Read the model definition and answer for the solid it produces. Units are mm, in the model's axes. Round coordinates to 2 decimals unless told otherwise and drop trailing zeros. Write each loop counter-clockwise with the first axis right and the second up, starting at its lowest first coordinate (ties: lowest second). Pieces come first, ordered by that corner, then holes.
from build123d import *

# Parameters (mm, degrees)
F0_W            = 139.7
F0_H            = 3.175
F1_DEPTH        = 50.8
F3_D            = 3.3
F4_W            = 38.1
F4_H            = 38.1
F5_DEPTH        = 3.176
F7_D            = 2.2606
F9_D            = 2.7051
F11_D           = 2.2606
F13_D           = 4.9784
F13_CSINK_D     = 9.1186
F13_CSINK_ANGLE = 82


with BuildPart() as f1:
    # F0 (on Front) → F1 (new body, symmetric)
    with BuildSketch(Plane.XZ):
        with Locations((-69.85, 1.5875)):
            Rectangle(F0_W, F0_H)
    extrude(amount=F1_DEPTH, both=True)

    # F3 (through all)
    with Locations(Plane.XY.offset(3.175)):
        with Locations((-78.994, 4.572), (-78.994, -4.572), (-89.154, 0), (-109.22, 0), (-119.38, 4.572), (-119.38, -4.572)):
            Hole(F3_D / 2)

    # F4 (on face) → F5 (cut, through all)
    with BuildSketch(Plane.XY.offset(3.175)):
        with Locations((-19.05, 31.75)):
            Rectangle(F4_W, F4_H)
    extrude(amount=-F5_DEPTH, mode=Mode.SUBTRACT)

    # F7 (through all)
    with Locations(Plane.XY.offset(3.175)):
        with Locations((-26.9875, -44.45), (-26.9875, -19.05), (-4.7625, -19.05), (-4.7625, -44.45)):
            Hole(F7_D / 2)

    # F9 (through all)
    with Locations(Plane.XY.offset(3.175)):
        with Locations((-86.36, 11.43), (-66.36, 11.43)):
            Hole(F9_D / 2)

    # F11 (through all)
    with Locations(Plane.XY.offset(3.175)):
        with Locations((-135.382, -2.54), (-98.298, -2.54), (-98.298, 22.225), (-135.382, 22.225)):
            Hole(F11_D / 2)

    # F13 (through all)
    with Locations(Plane(origin=(0, 0, 0), x_dir=(1, 0, 0), z_dir=(0, 0, -1))):
        with Locations((-30.1625, 31.75)):
            CounterSinkHole(F13_D / 2, F13_CSINK_D / 2, counter_sink_angle=F13_CSINK_ANGLE)


solid = f1.part
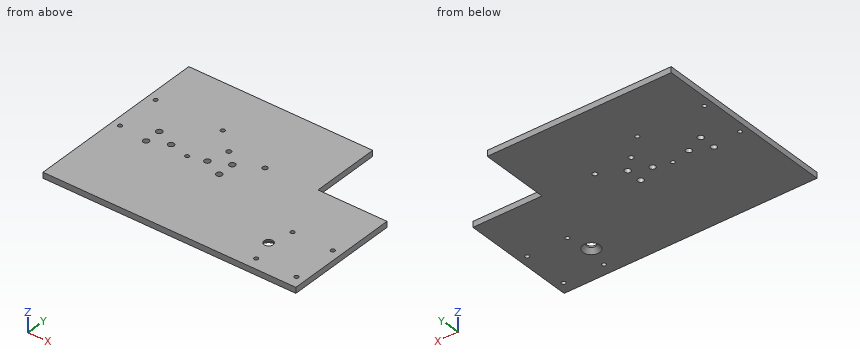
Q1. Section D-D (z = 0.7) is taken. State how many separate pieces and enclosed holes the cut face has, then the cut area to 3 significant figures.
Verdict:
separate pieces: 1
enclosed holes: 17
area: 12,600 mm2
Q2. Straight lines are drawn through the part: probe 1 along X at (y, z) = (22.5, 1.45); probe 2 along X at (y, z) = (-1, 2.1); probe 3 along Y at (x, z) = (-24.5, 1.85). For each, find the intervals that lie inside material, in ascending order.
Verdict:
probe 1: x = -139.7 to -136.48, -134.29 to -99.39, -97.2 to -38.1
probe 2: x = -139.7 to -110.53, -107.91 to -90.47, -87.84 to 0
probe 3: y = -50.8 to 12.7
Q3. Flat-ended cylindrical pins translate along their axes: pin 1 Ø2 at (x, y) = (-119.38, 4.572) entering from +Z; pin 2 Ø5.5 at (x, y) = (-89.154, 0) entering from -Z. Find the tip coordinate at first contact, or state that the pin passes through.
Verdict:
pin 1: passes through
pin 2: stops at z = 0
Q4. Section B-B (x = -109.22) is taken. Determine the outline of the cut face in (y, z) (3 decimals), then the cut area to 3 significant figures.
Verdict:
outline: (-50.8, 0) - (-1.65, 0) - (-1.65, 3.175) - (-50.8, 3.175) - close; (1.65, 0) - (50.8, 0) - (50.8, 3.175) - (1.65, 3.175) - close
area: 312 mm2
Q5. Section C-C (y = 0) is taken. Determine the outline of the cut face in (x, z) (3 decimals).
Verdict:
outline: (-139.7, 0) - (-110.87, 0) - (-110.87, 3.175) - (-139.7, 3.175) - close; (-107.57, 0) - (-90.804, 0) - (-90.804, 3.175) - (-107.57, 3.175) - close; (-87.504, 0) - (0, 0) - (0, 3.175) - (-87.504, 3.175) - close
Q6. Section A-A (y = -31.75) is taken. Determine the outline of the cut face in (x, z) (3 decimals), then the cut area to 3 significant figures.
Verdict:
outline: (-139.7, 0) - (-34.722, 0) - (-32.652, 2.381) - (-32.652, 3.175) - (-139.7, 3.175) - close; (-27.673, 2.381) - (-25.603, 0) - (0, 0) - (0, 3.175) - (-27.673, 3.175) - close
area: 423 mm2
